The drawing under review shows one solid part. Ordinate dimensions are in mm from its lowest x, y, z. Coordinates: 2 decimals unless noted, no trailing zeros. Loops run counter-clockwise (first coordinate to the right, second up) from the corner with the lowest first, then second, coordinate; pieces in that order, holes last. Notation, with made-up numbers: (-31.75, -23.5) - (-2.75, -23.5) arc R24 cw to (-2.75, 13.5) - close; hole circle Ø3 at (-14.5, -29.5). An arc over 180 degrees is marked (long way). Answer as a JSON object with one key per item and string values. Group by question number.
Item 1: We need section C-C (z = 0.6). Give the boundary of the cut face in (x, y) (1 decimal), then the cut area to 3 significant figures.
Item 2: To check wall thickness, follow line 1 (X direction, y = 6.5, z = 0.6); line 2 (X direction, y = 12, z = 0.6); line 3 (Y direction, x = 35, z = 1.5) (1 decimal). State the ranges of each line that lie inside material, in increasing order.
Item 3: We need section A-A (y = 7.25). Give the boundary of the cut face in (x, z).
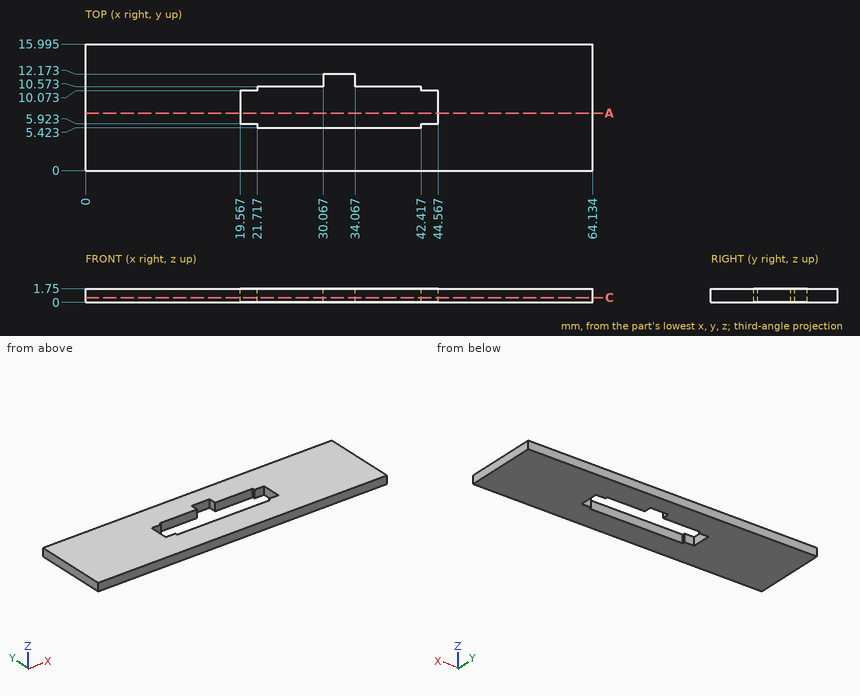
Check sheet entries:
{
 "1": {"outline": "(0, 0) - (64.1, 0) - (64.1, 16) - (0, 16) - close; hole (19.6, 5.9) - (21.7, 5.9) - (21.7, 5.4) - (42.4, 5.4) - (42.4, 5.9) - (44.6, 5.9) - (44.6, 10.1) - (42.4, 10.1) - (42.4, 10.6) - (34.1, 10.6) - (34.1, 12.2) - (30.1, 12.2) - (30.1, 10.6) - (21.7, 10.6) - (21.7, 10.1) - (19.6, 10.1) - close", "area": "895 mm2"},
 "2": {"line 1": "x = 0 to 19.57, 44.57 to 64.13", "line 2": "x = 0 to 30.07, 34.07 to 64.13", "line 3": "y = 0 to 5.4, 10.6 to 16"},
 "3": {"outline": "(0, 0) - (19.57, 0) - (19.57, 1.75) - (0, 1.75) - close; (44.57, 0) - (64.13, 0) - (64.13, 1.75) - (44.57, 1.75) - close"}
}
